Geometry check sheet. Reference: the model listing, model coordinates, mm. Face numbers are marked on the shaded views. Give positions to 0.01 mm unless a question says otherwise; leave off trailing zeros. Loops run counter-clockwise (first coordinate to the right, second up) from the corner with the lowest first, then second, coordinate; pieces in that order, holes last. Notation, with made-up numbers: (59, 64.5) -> (96, 64.5) arc R19 ccw to (96, 92.5) -> close; hole circle Ø1 at (16.25, 29.25). An arc over 180 degrees is marked (long way). One line per question, with ' | ' between items.
from build123d import *

# Parameters (mm, degrees)
F0_W        = 100
F0_H        = 50
F1_DEPTH    = 25
F2_R        = 15
F3_DEPTH    = 25.001
F4_R        = 5
F5_T1_DEPTH = 32.5
F5_S5_W     = 5
F5_S5_H     = 5
F5_T6_DEPTH = 5
F6_T1_DEPTH = 32.5
F6_S5_W     = 5
F6_S5_H     = 5
F6_T6_DEPTH = 5


# Not quite as in the source:
# - a fillet or chamfer that OpenCascade refuses, or shapes differently, is made with other operations: its cross-section is extruded or revolved along the edge and cut away or added


with BuildPart() as f1:
    # F0 (on Top) → F1 (new body)
    with BuildSketch(Plane.XY):
        Rectangle(F0_W, F0_H)
    extrude(amount=F1_DEPTH)

    # F2 (on face) → F3 (cut, through all)
    with BuildSketch(Plane.XY.offset(25)):
        Circle(F2_R)
    extrude(amount=-F3_DEPTH, mode=Mode.SUBTRACT)

    # F4
    f4_edges = [f1.edges().sort_by_distance(p)[0] for p in [
        (0, 25, 25),
        (-50, 0, 25),
        (-50, -25, 12.5),
        (50, -25, 12.5),
        (0, -25, 0),
        (0, -25, 25),
        (50, 0, 25),
    ]]
    fillet(f4_edges, radius=F4_R)

    # F5: fillet of radius 5 on 1 edges, made by hand

    # F5_s2 → F5_t1 (cut)
    with BuildSketch(Plane.XY.offset(-12.5)):
        with BuildLine():
            ThreePointArc((-50, 20), (-48.5355339059, 23.5355339059), (-45, 25))
            Line((-45, 25), (-50, 25))
            Line((-50, 25), (-50, 20))
        make_face()
    extrude(amount=F5_T1_DEPTH, mode=Mode.SUBTRACT)


with BuildPart() as f5_tool4:
    # F5_s5 → F5_t6 (new body)
    with BuildSketch(Plane.YZ.offset(-45)):
        with Locations((22.5, 22.5)):
            Rectangle(F5_S5_W, F5_S5_H)
    extrude(amount=-F5_T6_DEPTH)

    # F5_s7 → F5_t8 (revolve, cut)
    with BuildSketch(Plane(origin=(-45, 20, 20), x_dir=(0, -0.7071067812, -0.7071067812), z_dir=(0, 0.7071067812, -0.7071067812))):
        with BuildLine():
            ThreePointArc((0, -5), (5, 0), (0, 5))
            Line((0, 5), (0, -5))
        make_face()
    revolve(axis=Axis((-45, 20, 20), (-1, 0, 0)), mode=Mode.SUBTRACT)


with BuildPart() as f1_1:
    add(f1.part)

    # F5_t3: cut F5_tool4
    add(f5_tool4.part, mode=Mode.SUBTRACT)

    # F6: fillet of radius 5 on 1 edges, made by hand

    # F6_s2 → F6_t1 (cut)
    with BuildSketch(Plane.XY.offset(-12.5)):
        with BuildLine():
            ThreePointArc((45, 25), (48.5355339059, 23.5355339059), (50, 20))
            Line((50, 20), (50, 25))
            Line((50, 25), (45, 25))
        make_face()
    extrude(amount=F6_T1_DEPTH, mode=Mode.SUBTRACT)


with BuildPart() as f6_tool4:
    # F6_s5 → F6_t6 (new body)
    with BuildSketch(Plane.XZ.offset(-20)):
        with Locations((47.5, 22.5)):
            Rectangle(F6_S5_W, F6_S5_H)
    extrude(amount=-F6_T6_DEPTH)

    # F6_s7 → F6_t8 (revolve, cut)
    with BuildSketch(Plane(origin=(45, 20, 20), x_dir=(-0.7071067812, 0, -0.7071067812), z_dir=(0.7071067812, 0, -0.7071067812))):
        with BuildLine():
            ThreePointArc((0, -5), (5, 0), (0, 5))
            Line((0, 5), (0, -5))
        make_face()
    revolve(axis=Axis((45, 20, 20), (0, 1, 0)), mode=Mode.SUBTRACT)


with BuildPart() as f1_2:
    add(f1_1.part)

    # F6_t3: cut F6_tool4
    add(f6_tool4.part, mode=Mode.SUBTRACT)


solid = f1_2.part
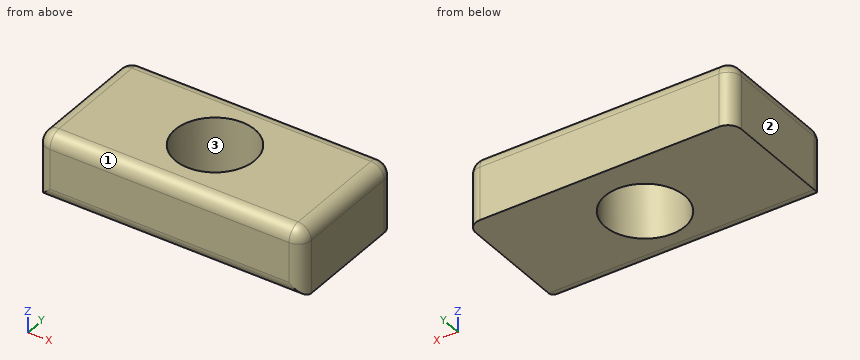
Item 1: Sectioned sample at D-D (y = 8.5). Record the cut outline in (x, z).
Result:
outline: (-50, 0) -> (-12.36, 0) -> (-12.36, 25) -> (-45, 25) arc R5 ccw to (-50, 20) -> close; (12.36, 0) -> (50, 0) -> (50, 20) arc R5 ccw to (45, 25) -> (12.36, 25) -> close
Item 2: Release check for a two-part mould opening along X. For the marked faces 1, 2 and 3 record: pulls with the +X half, pulls with the -X half, needs draft (parallel to the pull), parting line crosses it, or undercut.
Result:
face 1: needs draft | face 2: pulls with the -X half | face 3: undercut
Item 3: Sectioned sample at A-A (y = 0). Record the cut outline in (x, z), plus the area to 3 significant figures.
Result:
outline: (-50, 0) -> (-15, 0) -> (-15, 25) -> (-45, 25) arc R5 ccw to (-50, 20) -> close; (15, 0) -> (50, 0) -> (50, 20) arc R5 ccw to (45, 25) -> (15, 25) -> close | area: 1,740 mm2
Item 4: Sectioned sample at B-B (x = 12). Record the cut outline in (y, z), plus the area to 3 significant figures.
Result:
outline: (-25, 5) arc R5 ccw to (-20, 0) -> (-9, 0) -> (-9, 25) -> (-20, 25) arc R5 ccw to (-25, 20) -> close; (9, 0) -> (25, 0) -> (25, 20) arc R5 ccw to (20, 25) -> (9, 25) -> close | area: 784 mm2
Item 5: Sectioned sample at C-C (x = 0). Record the cut outline in (y, z), plus the area to 3 significant figures.
Result:
outline: (-25, 5) arc R5 ccw to (-20, 0) -> (-15, 0) -> (-15, 25) -> (-20, 25) arc R5 ccw to (-25, 20) -> close; (15, 0) -> (25, 0) -> (25, 20) arc R5 ccw to (20, 25) -> (15, 25) -> close | area: 484 mm2
Item 6: Depth check by flat-ended pin: pin 1 Ø1.5 at (x, z) = (-30, 21.5) entering from -Y. Enter the tip coordinate at first touch or a pass-through.
Result:
pin 1: y = -24.94
Item 7: Scan lines: probe 1 along Y at (x, z) = (0, 19); probe 2 along X at (y, z) = (7.5, 10); probe 3 along X at (y, z) = (-12, 5.5). Record each from-to range of solid material in increasing order.
Result:
probe 1: -25 to -15, 15 to 25 | probe 2: -50 to -12.99, 12.99 to 50 | probe 3: -50 to -9, 9 to 50
